```python
from build123d import *

# Parameters (mm, degrees)
F1_DEPTH = 2


with BuildPart() as f1:
    # F0 (on Top) → F1 (new body)
    with BuildSketch(Plane.XY):
        with BuildLine():
            ThreePointArc((-18.525, 9.79253), (-19.58566, 9.35319), (-20.025, 8.29253))
            Line((-20.025, 8.29253), (-20.025, -4.00747))
            Line((-20.025, -4.00747), (-17.025, -4.00747))
            Line((-17.025, -4.00747), (-17.025, 8.29253))
            ThreePointArc((-17.025, 8.29253), (-17.46434, 9.35319), (-18.525, 9.79253))
        make_face()
        with BuildLine():
            Line((20.475, 9.79253), (-18.525, 9.79253))
            ThreePointArc((-18.525, 9.79253), (-17.46434, 9.35319), (-17.025, 8.29253))
            Line((-17.025, 8.29253), (-17.025, -4.00747))
            Line((-17.025, -4.00747), (-17.025, -8.50747))
            ThreePointArc((-17.025, -8.50747), (-17.46434, -9.56813), (-18.525, -10.00747))
            Line((-18.525, -10.00747), (20.475, -10.00747))
            ThreePointArc((20.475, -10.00747), (19.41434, -9.56813), (18.975, -8.50747))
            Line((18.975, -8.50747), (18.975, 3.79253))
            Line((18.975, 3.79253), (18.975, 8.29253))
            ThreePointArc((18.975, 8.29253), (19.41434, 9.35319), (20.475, 9.79253))
        make_face()
        with BuildLine():
            ThreePointArc((-11.525, 1.89253), (-10.64632, 4.01385), (-8.525, 4.89253))
            Line((-8.525, 4.89253), (10.475, 4.89253))
            ThreePointArc((10.475, 4.89253), (12.59632, 4.01385), (13.475, 1.89253))
            Line((13.475, 1.89253), (13.475, -2.10747))
            ThreePointArc((13.475, -2.10747), (12.59632, -4.22879), (10.475, -5.10747))
            Line((10.475, -5.10747), (-8.525, -5.10747))
            ThreePointArc((-8.525, -5.10747), (-10.64632, -4.22879), (-11.525, -2.10747))
            Line((-11.525, -2.10747), (-11.525, 1.89253))
        make_face(mode=Mode.SUBTRACT)
        with BuildLine():
            ThreePointArc((18.975, -8.50747), (19.41434, -9.56813), (20.475, -10.00747))
            ThreePointArc((20.475, -10.00747), (21.53566, -9.56813), (21.975, -8.50747))
            Line((21.975, -8.50747), (21.975, 3.79253))
            Line((21.975, 3.79253), (18.975, 3.79253))
            Line((18.975, 3.79253), (18.975, -8.50747))
        make_face()
    extrude(amount=F1_DEPTH)


solid = f1.part
```
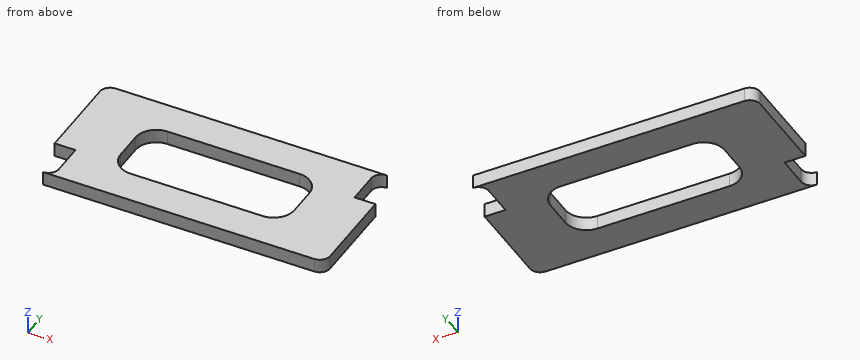
Build history of the part. All positions in model axes, mm. Give positions to 0.01 mm unless a question says otherwise; leave off trailing zeros. Order: outer loops, then holes, each group sorted by start corner. A loop starts at its lowest first (then second) coordinate and runs counter-clockwise, first axis right, second up. Notation, with made-up numbers: M 28.5,-1 L 36.5,-1 A35 ccw 36.5,33 Z; hole C 67.25,61 d10. An arc over 180 degrees is marked long. Return JSON: item names as keys, results as strings.
Q1. Band-saw the part on C-C (y = -3.5). Give the cut face in (x, z) (3 decimals), then the cut area to 3 significant figures.
Answer list:
{"outline": "M -20.025,0 L -11.182,0 L -11.182,2 L -20.025,2 Z; M 13.132,0 L 21.975,0 L 21.975,2 L 13.132,2 Z", "area": "35.4 mm^2"}
Q2. Band-saw the part on A-A (x = 5). Give the cut face in (y, z), then the cut area to 3 significant figures.
Answer list:
{"outline": "M -10.01,0 L -5.11,0 L -5.11,2 L -10.01,2 Z; M 4.89,0 L 9.79,0 L 9.79,2 L 4.89,2 Z", "area": "19.6 mm^2"}
Q3. Band-saw the part on D-D (y = -7.75). Give the cut face in (x, z) (3 decimals), then the cut area to 3 significant figures.
Answer list:
{"outline": "M -17.025,0 L 21.975,0 L 21.975,2 L -17.025,2 Z", "area": "78.0 mm^2"}
Q4. Wall check: probe 1 along Y at (x, z) = (-8, 0.35); probe 2 along X at (y, z) = (0, 0.3) (3 decimals); probe 3 along X at (y, z) = (-8.25, 0.3) (3 decimals). Give the ranges that are in metal, low to high. Write a range as from..to.
Answer list:
{"probe 1": "y = -10.01..-5.11, 4.89..9.79", "probe 2": "x = -20.025..-11.525, 13.475..21.975", "probe 3": "x = -17.025..21.975"}
Q5. Band-saw the part on B-B (z = 1.5). Give the cut face in (x, y) (3 decimals).
Answer list:
{"outline": "M -20.025,-4.007 L -17.025,-4.007 L -17.025,-8.507 A1.5 cw -18.525,-10.007 L 20.475,-10.007 A1.5 ccw 21.975,-8.507 L 21.975,3.793 L 18.975,3.793 L 18.975,8.293 A1.5 cw 20.475,9.793 L -18.525,9.793 A1.5 ccw -20.025,8.293 Z; hole M -11.525,-2.107 A3 ccw -8.525,-5.107 L 10.475,-5.107 A3 ccw 13.475,-2.107 L 13.475,1.893 A3 ccw 10.475,4.893 L -8.525,4.893 A3 ccw -11.525,1.893 Z"}
